from build123d import *

# Parameters (mm, degrees)
SALIENTE_EXTRUIR1_DEPTH = 11
CROQUIS13_W             = 3
CROQUIS13_H             = 12
SALIENTE_EXTRUIR3_DEPTH = 11.044424957
CROQUIS15_W             = 13
CROQUIS15_H             = 3.3
SALIENTE_EXTRUIR5_DEPTH = 11
REDONDEO1_RADIUS        = 5.522212479
REDONDEO1_LENGTH        = 3
REDONDEO2_RADIUS        = 5.5
REDONDEO2_LENGTH        = 3.3
REDONDEO3_RADIUS        = 5.5
REDONDEO3_LENGTH        = 3.3
CROQUIS16_R             = 1.6
CORTAR_EXTRUIR6_DEPTH   = 54.876956991
CROQUIS17_R             = 1.6
CORTAR_EXTRUIR7_DEPTH   = 55.423216504


with BuildPart() as part:
    # Croquis2 → Saliente-Extruir1 (new body)
    with BuildSketch(Plane.XY):
        Polygon((-7.377824178, -34.958999634), (10.003000259, -34.958999634), (10.003000259, -45.958999634), (-11.996999741, -45.958999634), (-21.032533647, -36.923465728), (-13.222945865, -29.113877947), align=None)
    extrude(amount=SALIENTE_EXTRUIR1_DEPTH)

    # Croquis13 → Saliente-Extruir3 (add)
    with BuildSketch(Plane(origin=(-21.168411906, -21.168411906, 0), x_dir=(0, 0, -1), z_dir=(0.7071067811865442, 0.7071067811865508, 0))):
        with Locations((-5.5, -5.236585834)):
            Rectangle(CROQUIS13_W, CROQUIS13_H)
    extrude(amount=-SALIENTE_EXTRUIR3_DEPTH)

    # Croquis15 → Saliente-Extruir5 (add, through all)
    with BuildSketch(Plane(origin=(0, -34.958999634, 0), x_dir=(1, 0, 0), z_dir=(0, 1, 0))):
        with Locations((16.503000259, -2.25)):
            Rectangle(CROQUIS15_W, CROQUIS15_H)
        with Locations((16.503000259, -8.75)):
            Rectangle(CROQUIS15_W, CROQUIS15_H)
    extrude(amount=-SALIENTE_EXTRUIR5_DEPTH)

    # Redondeo1: full round fillet: the end face becomes a half cylinder, R = half its width
    redondeo1_face = Plane((-25.61302113, -24.533390463, 5.5), x_dir=(0, 0, -1), z_dir=(-0.707106781187, 0.707106781187, 0))  # on the end face: x along it, z out of the body
    redondeo1_slab = redondeo1_face.offset(-REDONDEO1_RADIUS / 2) * Box(REDONDEO1_LENGTH, 2 * REDONDEO1_RADIUS, REDONDEO1_RADIUS, mode=Mode.PRIVATE)  # the body's end, R deep
    redondeo1_round = Plane((-21.708227239, -28.438184354, 5.5), x_dir=(-0.707106781187, 0.707106781187, 0), z_dir=(0, 0, -1)) * Cylinder(REDONDEO1_RADIUS, REDONDEO1_LENGTH, mode=Mode.PRIVATE)  # its axis R under the face
    add(redondeo1_slab - redondeo1_round, mode=Mode.SUBTRACT)

    # Redondeo2: full round fillet: the end face becomes a half cylinder, R = half its width
    redondeo2_face = Plane((23.003000259, -40.458999634, 8.75), x_dir=(0, 0, -1), z_dir=(1, 0, 0))  # on the end face: x along it, z out of the body
    redondeo2_slab = redondeo2_face.offset(-REDONDEO2_RADIUS / 2) * Box(REDONDEO2_LENGTH, 2 * REDONDEO2_RADIUS, REDONDEO2_RADIUS, mode=Mode.PRIVATE)  # the body's end, R deep
    redondeo2_round = Plane((17.503000259, -40.458999634, 8.75), x_dir=(1, 0, 0), z_dir=(0, 0, -1)) * Cylinder(REDONDEO2_RADIUS, REDONDEO2_LENGTH, mode=Mode.PRIVATE)  # its axis R under the face
    add(redondeo2_slab - redondeo2_round, mode=Mode.SUBTRACT)

    # Redondeo3: full round fillet: the end face becomes a half cylinder, R = half its width
    redondeo3_face = Plane((23.003000259, -40.458999634, 2.25), x_dir=(0, 0, -1), z_dir=(1, 0, 0))  # on the end face: x along it, z out of the body
    redondeo3_slab = redondeo3_face.offset(-REDONDEO3_RADIUS / 2) * Box(REDONDEO3_LENGTH, 2 * REDONDEO3_RADIUS, REDONDEO3_RADIUS, mode=Mode.PRIVATE)  # the body's end, R deep
    redondeo3_round = Plane((17.503000259, -40.458999634, 2.25), x_dir=(1, 0, 0), z_dir=(0, 0, -1)) * Cylinder(REDONDEO3_RADIUS, REDONDEO3_LENGTH, mode=Mode.PRIVATE)  # its axis R under the face
    add(redondeo3_slab - redondeo3_round, mode=Mode.SUBTRACT)

    # Croquis16 → Cortar-Extruir6 (cut, through all)
    with BuildSketch(Plane(origin=(0, 0, 4), x_dir=(-1, 0, 0), z_dir=(0, 0, -1))):
        with Locations((21.70822724, -28.438184354)):
            Circle(CROQUIS16_R)
    extrude(amount=-CORTAR_EXTRUIR6_DEPTH, mode=Mode.SUBTRACT)

    # Croquis17 → Cortar-Extruir7 (cut, through all)
    with BuildSketch(Plane(origin=(0, 0, 0.6), x_dir=(-1, 0, 0), z_dir=(0, 0, -1))):
        with Locations((-17.503000259, -40.458999634)):
            Circle(CROQUIS17_R)
    extrude(amount=-CORTAR_EXTRUIR7_DEPTH, mode=Mode.SUBTRACT)


solid = part.part
Here's how the part is built. I have some questions about the finished solid (model axes, mm). A direction names the side the tool comes from. Coordinates: 2 decimals unless noted, no trailing zeros. Loops run counter-clockwise (first coordinate to the right, second up) from the corner with the lowest first, then second, coordinate; pieces in that order, holes last.
1. For P1, Ø0.7, axis at y = -43, z = 10.5, coming from the +X side; P2, Ø9, axis at x = 19.5, y = -38, coming from the -Z side; P3, Ø2, axis at y = -34.5, z = 5.5, coming from the -X side; P4, Ø1.9, axis at x = 17.503, y = -40.459, coming from the +Z side, each with a flat end and sliding along its axis, tell me the tip position at first contact or that it passes through.
2. Imagine slicing it at A-A, the plane x = 14. Please give me the cut outline in (y, z).
3. I need wall thicknesses on L1, parallel to Y at x = 4, z = 6.75; L2, parallel to Z at x = -16.5, y = -26.75; L3, parallel to Y at x = -12, z = 2.25. Which ranges of each line are inside material? Lowest first, please.
4. If we mould it in two halves opening along Y, with no side actions, what happens to faces 1 (the cylindrical face through (-25.7, -24.62, 5.48)), 2 (the cylindrical face through (-22.57, -27.09, 5.48)), 3 (the flat face through (-20, -30, 4))? For each: pulls with the +Y half, pulls with the -Y half, needs draft (parallel to the pull), parting line crosses it, or undercut.
5. Imagine slicing it at B-B, the plane z = 2. Please give me the cut outline in (x, y).
6. Imagine slicing it at C-C, the plane y = -36.25. Please give me the cut outline in (x, z), and give its area (3 significant figures).
7. Imagine slicing it at D-D, the plane x = 1. Please give me the cut outline in (y, z).
8. For faces 4 (the flat face through (15, -40, 0.6)), 5 (the flat face through (-17.18, -33.07, 1.97)), 6 (the flat face through (15, -40, 3.9)), which set-ups out of +Z, -Z, +X, -X, +Y, -Y let a thin tool reach every point of the face, with its end or its side?
Taken from the geometry:
1. P1: stops at x = 22.54
1. P2: stops at z = 0.6
1. P3: stops at x = -24.46
1. P4: passes through
2. outline: (-45.96, 0.6) - (-34.96, 0.6) - (-34.96, 3.9) - (-45.96, 3.9) - close; (-45.96, 7.1) - (-34.96, 7.1) - (-34.96, 10.4) - (-45.96, 10.4) - close
3. L1: y = -45.96 to -34.96
3. L2: z = 4 to 7
3. L3: y = -45.96 to -30.34
4. face 1: parting line crosses it
4. face 2: undercut
4. face 3: needs draft
5. outline: (-21.03, -36.92) - (-12, -45.96) - (17.5, -45.96) arc R5.5 ccw to (17.5, -34.96) - (-7.38, -34.96) - (-13.22, -29.11) - close; hole circle Ø3.2 at (17.5, -40.46)
6. outline: (-21.71, 4) - (-20.36, 4) - (-20.36, 0) - (10, 0) - (10, 0.6) - (21.04, 0.6) - (21.04, 3.9) - (10, 3.9) - (10, 7.1) - (21.04, 7.1) - (21.04, 10.4) - (10, 10.4) - (10, 11) - (-20.36, 11) - (-20.36, 7) - (-21.71, 7) - close
6. area: 411 mm2
7. outline: (-45.96, 0) - (-34.96, 0) - (-34.96, 11) - (-45.96, 11) - close
8. face 4: -Z, +X, +Y, -Y
8. face 5: -Z, -X, +Y
8. face 6: +X, +Y, -Y
